from build123d import *

# Parameters (mm, degrees)
SKETCH_4_W      = 57
SKETCH_4_H      = 145
EXTRUDE_1_DEPTH = 2
SKETCH_5_W      = 7.875
SKETCH_5_H      = 2
EXTRUDE_2_DEPTH = 2
SKETCH_6_W      = 21
SKETCH_6_H      = 2
EXTRUDE_3_DEPTH = 2
EXTRUDE_START   = -57
SKETCH_6_2_W    = 21
SKETCH_6_2_H    = 2
EXTRUDE_4_DEPTH = 4
EXTRUDE_START_2 = -2.2
EXTRUDE_5_DEPTH = 142.8


with BuildPart() as part:
    # 草图4 → 凸台-拉伸1 (new body)
    with BuildSketch(Plane(origin=(0, 0, 0), x_dir=(1, 0, 0), z_dir=(0, 1, 0))):
        Rectangle(SKETCH_4_W, SKETCH_4_H)
    extrude(amount=EXTRUDE_1_DEPTH)

    # 草图5 → 凸台-拉伸2 (add)
    with BuildSketch(Plane(origin=(0, 0, -72.5), x_dir=(-1, 0, 0), z_dir=(0, 0, -1))):
        with Locations((-24.5625, 1)):
            Rectangle(SKETCH_5_W, SKETCH_5_H)
        with Locations((-8.1875, 1)):
            Rectangle(SKETCH_5_W, SKETCH_5_H)
        with Locations((8.1875, 1)):
            Rectangle(SKETCH_5_W, SKETCH_5_H)
        with Locations((24.5625, 1)):
            Rectangle(SKETCH_5_W, SKETCH_5_H)
    extrude(amount=EXTRUDE_2_DEPTH)

    # 草图6 → 凸台-拉伸3 (add)
    with BuildSketch(Plane.ZY.offset(28.5)):
        with Locations((-43, 1)):
            Rectangle(SKETCH_6_W, SKETCH_6_H)
        with Locations((-1, 1)):
            Rectangle(SKETCH_6_W, SKETCH_6_H)
        with Locations((41, 1)):
            Rectangle(SKETCH_6_W, SKETCH_6_H)
    extrude(amount=EXTRUDE_3_DEPTH)

    # 草图6<2> → 凸台-拉伸4 (add)
    with BuildSketch(Plane.ZY.offset(28.5).offset(EXTRUDE_START)):
        with Locations((-43, 1)):
            Rectangle(SKETCH_6_2_W, SKETCH_6_2_H)
        with Locations((-1, 1)):
            Rectangle(SKETCH_6_2_W, SKETCH_6_2_H)
        with Locations((41, 1)):
            Rectangle(SKETCH_6_2_W, SKETCH_6_2_H)
    extrude(amount=-EXTRUDE_4_DEPTH)

    # 草图8 → 凸台-拉伸5 (add)
    with BuildSketch(Plane.XY.offset(72.5).offset(EXTRUDE_START_2)):
        Polygon((-11.6, 3.8), (-9.8, 2), (9.8, 2), (11.6, 3.8), (9.8, 3.8), (-9.8, 3.8), align=None)
    extrude(amount=-EXTRUDE_5_DEPTH)


solid = part.part
Verification items for the finished model (mm, model axes). Give positions to 0.01 mm unless a question says otherwise; leave off trailing zeros. Loops run counter-clockwise (first coordinate to the right, second up) from the corner with the lowest first, then second, coordinate; pieces in that order, holes last.
1) Draft check along X on faces 1 (the flat face through (0, 2, -72.5)), 2 (the flat face through (-13, 2, 0)). Enter one of: pulls with the +X half, pulls with the -X half, needs draft (parallel to the pull), parting line crosses it, or undercut.
2) Thickness scan on line 1 along Y through (x, z) = (17, -14.5); line 2 along Z through (x, y) = (15, 0.65); line 3 along Z through (x, y) = (-4, 2.8). Record the ranges inside material, lowest first.
3) Sectioned sample at C-C, the plane y = 3.2. Enter the section's corners in (x, z).
4) Sectioned sample at A-A, the plane z = -60. Enter the section's corners in (x, y), then the cut area to 3 significant figures.
5) Sectioned sample at B-B, the plane x = -16. Enter the section's corners in (y, z).
6) Depth check by flat-ended pin: pin 1 Ø1 at (y, z) = (1, -73.5) entering from +X; pin 2 Ø8 at (x, z) = (5.5, 48.5) entering from -Y; pin 3 Ø1 at (x, y) = (-17, 1) entering from -Z; pin 4 Ø0.5 at (x, y) = (-2, 2.5) entering from +Z. Enter the tip coordinate at first touch or a pass-through.
7) Sectioned sample at D-D, the plane z = 44.5. Enter the section's corners in (x, y).
Answers:
1. face 1: undercut
1. face 2: needs draft
2. line 1: y = 0 to 2
2. line 2: z = -72.5 to 72.5
2. line 3: z = -72.5 to 70.3
3. outline: (-11, -72.5) - (11, -72.5) - (11, 70.3) - (-11, 70.3) - close
4. outline: (-28.5, 0) - (28.5, 0) - (28.5, 2) - (9.8, 2) - (11.6, 3.8) - (-11.6, 3.8) - (-9.8, 2) - (-28.5, 2) - close
4. area: 153 mm2
5. outline: (0, -72.5) - (2, -72.5) - (2, 72.5) - (0, 72.5) - close
6. pin 1: stops at x = 28.5
6. pin 2: stops at y = 0
6. pin 3: stops at z = -72.5
6. pin 4: stops at z = 70.3
7. outline: (-30.5, 0) - (32.5, 0) - (32.5, 2) - (9.8, 2) - (11.6, 3.8) - (-11.6, 3.8) - (-9.8, 2) - (-30.5, 2) - close
